from build123d import *

# Parameters (mm, degrees)
SKETCH1_R           = 20
BOSS_EXTRUDE1_DEPTH = 50
SKETCH2_R           = 19
BOSS_EXTRUDE2_DEPTH = 20
SKETCH4_R           = 17.5
CUT_EXTRUDE1_DEPTH  = 40
SKETCH5_R           = 7.5
CUT_EXTRUDE2_DEPTH  = 5
SKETCH6_R           = 9
SKETCH6_R_2         = 7.5
BOSS_EXTRUDE3_DEPTH = 2


with BuildPart() as part:
    # Sketch1 → Boss-Extrude1 (new body)
    with BuildSketch(Plane.XY):
        Circle(SKETCH1_R)
    extrude(amount=BOSS_EXTRUDE1_DEPTH)

    # Sketch2 → Boss-Extrude2 (add, symmetric)
    with BuildSketch(Plane(origin=(0, 0, 0), x_dir=(0, 0, -1), z_dir=(1, 0, 0))):
        with Locations((-20, 0)):
            Circle(SKETCH2_R)
    extrude(amount=BOSS_EXTRUDE2_DEPTH, both=True)

    # Sketch4 → Cut-Extrude1 (cut)
    with BuildSketch(Plane(origin=(20, 0, 0), x_dir=(0, 0, -1), z_dir=(1, 0, 0))):
        with Locations((-20, 0)):
            Circle(SKETCH4_R)
    extrude(amount=-CUT_EXTRUDE1_DEPTH, mode=Mode.SUBTRACT)

    # Sketch5 → Cut-Extrude2 (cut)
    with BuildSketch(Plane.XY.offset(50)):
        Circle(SKETCH5_R)
    extrude(amount=-CUT_EXTRUDE2_DEPTH, mode=Mode.SUBTRACT)

    # Sketch6 → Boss-Extrude3 (add)
    with BuildSketch(Plane.XY.offset(50)):
        Circle(SKETCH6_R)
        Circle(SKETCH6_R_2, mode=Mode.SUBTRACT)
    extrude(amount=BOSS_EXTRUDE3_DEPTH)


solid = part.part
Could you check a few things on this model? Use its own coordinates, in mm. A direction names the side the tool comes from. Coordinates: 2 decimals unless noted, no trailing zeros. Order: outer loops, then holes, each group sorted by start corner. A loop starts at its lowest first (then second) coordinate and runs counter-clockwise, first axis right, second up.
Q1. Suppose I cut it at B-B on y = 3.5. Please give me the cut outline in (x, z).
Q2. Please list where these lines run through material, in increasing order: L1, parallel to Y at x = 0, z = 49; L2, parallel to Y at x = -6, z = 31; L3, parallel to Z at x = 6.5, y = 9.
Q3. Suppose I cut it at A-A on z = 20. Please give me the cut outline in (x, y) (3 decimals), and give its area (3 significant figures).
Q4. Which directions (+Z, -Z, +X, -X, +Y, -Y) give clear straight access to the entire face, cutting with the end or side of a thin tool? Please do faces 4 (the flat face through (0, 0, 45)), 5 (the cylindrical face through (15, -19, 20)), 6 (the cylindrical face through (-15, 19, 20)).
Q5. Suppose I cut it at C-C on x = 0. Please give me the cut outline in (y, z).
Q6. Suppose I cut it at D-D on z = 7. Please give me the cut outline in (x, y).
Q7. Thinking about a two-plate mould opening in Y: for faces 1 (the cylindrical face through (-7.493, 0.33, 48.451)), 2 (the cylindrical face through (-15, -19, 20)), 3 (the cylindrical face through (-4.336, -19.524, 30.206)), which applies, released by +Y, released by -Y, zero draft, split by the parting line, or undercut?
Q8. Will these pins go through, and if not, where does the flat tip stop? pin 1 (7.5 mm diameter, centred on x = 3, y = 2.5, fed in from +Z); pin 2 (1.5 mm diameter, centred on x = 14, z = 29, fed in from +Y); pin 3 (6 mm diameter, centred on x = 14.5, y = 9.5, fed in from +Z); pin 4 (8 mm diameter, centred on x = -12, z = 12, fed in from -Y).
Answer:
1. outline: (-20, 1.33) - (-19.69, 1.33) - (-19.69, 0) - (19.69, 0) - (19.69, 1.33) - (20, 1.33) - (20, 2.85) - (-20, 2.85) - close; (-20, 37.15) - (20, 37.15) - (20, 38.67) - (19.69, 38.67) - (19.69, 50) - (8.29, 50) - (8.29, 52) - (6.63, 52) - (6.63, 45) - (-6.63, 45) - (-6.63, 52) - (-8.29, 52) - (-8.29, 50) - (-19.69, 50) - (-19.69, 38.67) - (-20, 38.67) - close
2. L1: y = -20 to -7.5, 7.5 to 20
2. L2: y = -19.08 to -13.61, 13.61 to 19.08
2. L3: z = 0 to 4.99, 35.01 to 50
3. outline: (-20, -19) - (-6.245, -19) arc R20 ccw to (6.245, -19) - (20, -19) - (20, -17.5) - (-20, -17.5) - close; (-20, 17.5) - (20, 17.5) - (20, 19) - (6.245, 19) arc R20 ccw to (-6.245, 19) - (-20, 19) - close
3. area: 137 mm2
4. face 4: +Z
4. face 5: +X, -Y
4. face 6: -X, +Y
5. outline: (-20, 0) - (20, 0) - (20, 50) - (9, 50) - (9, 52) - (7.5, 52) - (7.5, 45) - (-7.5, 45) - (-7.5, 52) - (-9, 52) - (-9, 50) - (-20, 50) - close; hole circle Ø35 at (0, 20)
6. outline: (-20, -13.86) - (-14.42, -13.86) arc R20 ccw to (14.42, -13.86) - (20, -13.86) - (20, -11.72) - (-20, -11.72) - close; (-20, 11.72) - (20, 11.72) - (20, 13.86) - (14.42, 13.86) arc R20 ccw to (-14.42, 13.86) - (-20, 13.86) - close
7. face 1: undercut
7. face 2: released by -Y
7. face 3: split by the parting line
8. pin 1: stops at z = 52
8. pin 2: stops at y = 17.12
8. pin 3: stops at z = 50
8. pin 4: stops at y = -18.57
